from build123d import *

# Parameters (mm, degrees)
SKETCH1_R           = 12.7
BOSS_EXTRUDE1_DEPTH = 330.2
SKETCH3_R           = 12.7
SKETCH3_R_2         = 7.9375
CUT_EXTRUDE2_DEPTH  = 27.5336
SKETCH2_R           = 12.7
SKETCH2_R_2         = 7.9375
CUT_EXTRUDE1_DEPTH  = 13.7414
CHAMFER1_SIZE       = 1.27


with BuildPart() as part:
    # Sketch1 → Boss-Extrude1 (new body)
    with BuildSketch(Plane.XY):
        Circle(SKETCH1_R)
    extrude(amount=-BOSS_EXTRUDE1_DEPTH)

    # Sketch3 → Cut-Extrude2 (cut)
    with BuildSketch(Plane(origin=(0, 0, -330.2), x_dir=(-1, 0, 0), z_dir=(0, 0, -1))):
        Circle(SKETCH3_R)
        Circle(SKETCH3_R_2, mode=Mode.SUBTRACT)
    extrude(amount=-CUT_EXTRUDE2_DEPTH, mode=Mode.SUBTRACT)

    # Sketch2 → Cut-Extrude1 (cut)
    with BuildSketch(Plane.XY):
        Circle(SKETCH2_R)
        Circle(SKETCH2_R_2, mode=Mode.SUBTRACT)
    extrude(amount=-CUT_EXTRUDE1_DEPTH, mode=Mode.SUBTRACT)

    # Chamfer1
    chamfer1_edges = [part.edges().sort_by_distance(p)[0] for p in [
        (-7.9375, 0, 0),
        (7.9375, 0, -330.2),
    ]]
    chamfer(chamfer1_edges, length=CHAMFER1_SIZE)


solid = part.part
CAD build for the part. Positions are in the model's coordinates, mm. A direction names the side the tool comes from. Round coordinates to 2 decimals unless told otherwise and drop trailing zeros. Write each loop counter-clockwise with the first axis right and the second up, starting at its lowest first coordinate (ties: lowest second). Pieces come first, ordered by that corner, then holes. Notation, with made-up numbers: (-32, 65) -> (27, 65) arc R24 cw to (27, 87) -> close; hole circle Ø2 at (23.5, 79.25). An arc over 180 degrees is marked (long way). Answer as a JSON object with one key per item and string values.
(1) Band-saw the part on C-C, the plane z = -199. List the corners of the cut face in (x, y), then the cut area to 3 significant figures.
Reported:
{"outline": "circle Ø25.4 at (0, 0)", "area": "507 mm^2"}
(2) Pin check, flat tips, straight feed: P1, Ø1.5, axis at x = -6.5, z = -169.5, coming from the +Y side; P2, Ø8, axis at y = -8.5, z = -230.5, coming from the -X side; P3, Ø8, axis at x = 8, z = -60.5, coming from the +Y side; P4, Ø2, axis at y = -1, z = -89.5, coming from the +X side. Stop position of each tip, or through.
Reported:
{"P1": "stops at y = 11.32", "P2": "stops at x = -11.88", "P3": "stops at y = 12.05", "P4": "stops at x = 12.7"}
(3) Which spindle directions (+Z, -Z, +X, -X, +Y, -Y) get a long thin tool onto all of the face, cutting with end or side? Do faces 1 (the face through (-8.3, 0.2, -302.666)), 2 (the face through (-1.72, -7.75, -7.42)), 3 (the face through (0, 0, -330.2)). Say none if no direction does.
Reported:
{"face 1": "-Z", "face 2": "+Z", "face 3": "-Z, +X, -X, +Y, -Y"}
(4) Probe probe 1 along Y at (x, z) = (-1.25, -94); probe 2 along Z at (x, y) = (9, -8.25); probe 3 along X at (y, z) = (0.25, -110). List the from-to ranges inside material, lowest first. Write a range as [from, to].
Reported:
{"probe 1": "y = [-12.64, 12.64]", "probe 2": "z = [-302.67, -13.74]", "probe 3": "x = [-12.7, 12.7]"}
(5) Band-saw the part on A-A, the plane y = 0. List the corners of the cut face in (x, z).
Reported:
{"outline": "(-12.7, -302.67) -> (-7.94, -302.67) -> (-7.94, -328.93) -> (-6.67, -330.2) -> (6.67, -330.2) -> (7.94, -328.93) -> (7.94, -302.67) -> (12.7, -302.67) -> (12.7, -13.74) -> (7.94, -13.74) -> (7.94, -1.27) -> (6.67, 0) -> (-6.67, 0) -> (-7.94, -1.27) -> (-7.94, -13.74) -> (-12.7, -13.74) -> close"}
